Geometry check sheet. Reference: the model listing, model coordinates, mm. A direction names the side the tool comes from. Coordinates: 2 decimals unless noted, no trailing zeros. Order: outer loops, then holes, each group sorted by start corner. A loop starts at its lowest first (then second) coordinate and runs counter-clockwise, first axis right, second up. Notation, with made-up numbers: M -5,86.5 L 51,86.5 A21 ccw 51,93.5 Z; hole C 69.25,61 d1. An arc over 180 degrees is marked long. One line per item, written item: value. Start each with the question number.
1) Sectioned sample at B-B, the plane x = 311.5. Enter the section's corners in (y, z), then the cut area to 3 significant figures.
2) Thickness scan on L1, parallel to Y at x = 110.5, z = -65.5; L2, parallel to X at y = -310.5, z = -62.5; L3, parallel to Y at x = 813.5, z = -79.5. Record the ranges inside material, lowest first. Write a range as from..to.
3) Sectioned sample at C-C, the plane y = -520. Enter the section's corners in (x, z).
4) Sectioned sample at A-A, the plane z = -38. Enter the section's corners in (x, y).
5) Go/stop test with flat-tipped pins: P1, Ø3, axis at x = 295, z = -2.5, coming from the +Y side; P2, Ø5, axis at x = 519, y = -789.5, coming from the +Z side; P3, Ø2, axis at x = 657.5, y = -533, coming from the -Z side; P4, Ø8, axis at y = -744.5, z = -33, coming from the +X side. Record where each tip stops, or that it passes through.
6) Access from +Z, -Z, +X, -X, +Y, -Y to the whole of each face (thin tool, end or side, straight path). Record for faces 1 (the flat face through (19.05, -547, -53)), 2 (the cylindrical face through (976.46, -390.04, 3.76)), 3 (the flat face through (939, -374, 7.62)).
7) Sectioned sample at D-D, the plane x = 939.8. Enter the section's corners in (y, z).
8) Draft check along X on faces 4 (the flat face through (939, -76, 7.62)), 5 (the cylindrical face through (976.46, -91.4, 3.76)), 6 (the flat face through (706.9, -715.5, -43.8)), 7 (the flat face through (211, -996.95, -53)). Enter one of: pulls with the +X half, pulls with the -X half, needs draft (parallel to the pull), parting line crosses it, or undercut.
```python
from build123d import *

# Parameters (mm, degrees)
F1_DEPTH = 88.9
F2_DEPTH = 19.05
F3_R     = 39.6875
F4_DEPTH = 7.62


with BuildPart() as f1:
    # F0 (on Top) → F1 (new body)
    with BuildSketch(Plane.XY):
        Polygon((0, -76.2), (0, -1016), (406.4, -1016), (1016, -406.4), (1016, 0), (76.2, 0), align=None)
        Polygon((398.509232, -996.95), (19.05, -996.95), (19.05, -84.090768), (84.090768, -19.05), (996.95, -19.05), (996.95, -398.509232), align=None, mode=Mode.SUBTRACT)
    extrude(amount=-F1_DEPTH)

    # F0 (on Top) → F2 (join)
    with BuildSketch(Plane.XY):
        Polygon((19.05, -84.090768), (19.05, -996.95), (398.509232, -996.95), (996.95, -398.509232), (996.95, -19.05), (84.090768, -19.05), align=None)
    extrude(amount=-F2_DEPTH)

    # F3 (on face) → F4 (join)
    with BuildSketch(Plane.XY):
        with Locations((76.2, -939.8)):
            Circle(F3_R)
        with Locations((91.981537, -91.981537)):
            Circle(F3_R)
        with Locations((374.836927, -939.8)):
            Circle(F3_R)
        with Locations((939.8, -374.836927)):
            Circle(F3_R)
        with Locations((939.8, -76.2)):
            Circle(F3_R)
    extrude(amount=F4_DEPTH)


solid = f1.part
```
Final values:
1. outline: M -1016,-88.9 L -996.95,-88.9 L -996.95,-19.05 L -19.05,-19.05 L -19.05,-88.9 L 0,-88.9 L 0,0 L -1016,0 Z
1. area: 22,000 mm^2
2. L1: y = -1016..-996.95, -19.05..0
2. L2: x = 0..19.05, 996.95..1016
2. L3: y = -608.9..-581.96, -19.05..0
3. outline: M 0,-88.9 L 19.05,-88.9 L 19.05,-19.05 L 875.46,-19.05 L 875.46,-88.9 L 902.4,-88.9 L 902.4,0 L 0,0 Z
4. outline: M 0,-1016 L 406.4,-1016 L 1016,-406.4 L 1016,0 L 76.2,0 L 0,-76.2 Z; hole M 19.05,-996.95 L 398.51,-996.95 L 996.95,-398.51 L 996.95,-19.05 L 84.09,-19.05 L 19.05,-84.09 Z
5. P1: stops at y = 0
5. P2: stops at z = 0
5. P3: stops at z = -19.05
5. P4: stops at x = 681.9
6. face 1: -Z
6. face 2: +Z
6. face 3: +Z, +X, -X, +Y, -Y
7. outline: M -482.6,-88.9 L -455.66,-88.9 L -455.66,-19.05 L -19.05,-19.05 L -19.05,-88.9 L 0,-88.9 L 0,0 L -36.51,0 L -36.51,7.62 L -115.89,7.62 L -115.89,0 L -335.15,0 L -335.15,7.62 L -414.52,7.62 L -414.52,0 L -482.6,0 Z
8. face 4: needs draft
8. face 5: undercut
8. face 6: pulls with the +X half
8. face 7: undercut
